Check sheet for the modelled part. Datum: model origin and axes. Units: mm. A direction names the side the tool comes from. Coordinates: 2 decimals unless noted, no trailing zeros. Loops run counter-clockwise (first coordinate to the right, second up) from the corner with the lowest first, then second, coordinate; pieces in that order, holes last. Notation, with made-up numbers: M 80,30 L 87,30 A32 cw 87,64 Z; hole C 17,-38.5 d1. An arc over 180 degrees is marked long. Answer as CSV lines item,"result". Start each with the question number.
from build123d import *

# Parameters (mm, degrees)
CUT_EXTRUDE_1_DEPTH = 3
CHAMFER_1_SIZE      = 0.2


with BuildPart() as part:
    # 草图1 → 旋转1 (revolve)
    with BuildSketch(Plane.YZ, mode=Mode.PRIVATE) as revolve_1_sk:
        Polygon((0, 0), (-4.5, 0), (-4.5, -3.5), (-2.5, -3.5), (-2.5, -38.5), (-2, -38.5), (-2, -45.7), (0, -45.7), align=None)
    revolve(revolve_1_sk.sketch.rotate(Axis((0, 0, -45.7), (0, 0, 1)), 270), axis=Axis((0, 0, -45.7), (0, 0, 1)))

    # 草图2 → 切除-拉伸1 (cut)
    with BuildSketch(Plane.XY):
        Polygon((1.732050808, 0), (0.866025404, 1.5), (-0.866025404, 1.5), (-1.732050808, 0), (-0.866025404, -1.5), (0.866025404, -1.5), align=None)
    extrude(amount=-CUT_EXTRUDE_1_DEPTH, mode=Mode.SUBTRACT)

    # 倒角1
    chamfer_1_edges = [part.edges().sort_by_distance(p)[0] for p in [
        (4.5, 0, -3.5),
        (4.5, 0, 0),
    ]]
    chamfer(chamfer_1_edges, length=CHAMFER_1_SIZE)


solid = part.part
Item 1: Sectioned sample at A-A, the plane x = 0. Record the boundary of the cut face in (y, z), and give its area (3 significant figures).
Item 2: Release check for a two-part mould opening along Y. For faces 1 (the face through (-1.293, 0.76, -1.479)), 2 (the face through (0.54, 2.44, -21.24)), 3 (the face through (-2, 2, -3.5)) record: released by +Y, released by -Y, zero draft, split by the parting line, or undercut.
Item 3: Go/stop test with flat-tipped pins: pin 1 (2 mm diameter, centred on y = -0.5, z = -36.5, fed in from -X); pin 2 (1.5 mm diameter, centred on x = -0.5, y = -0.5, fed in from +Z); pin 3 (3 mm diameter, centred on y = -2.5, z = -29.5, fed in from +X). Record where each tip stops, or that it passes through.
Item 4: Sectioned sample at B-B, the plane z = -7. Record the boundary of the cut face in (x, y), and give its area (3 significant figures).
Item 5: Set-up check for faces 4 (the face through (0, 0, -45.7)), 5 (the face through (1, -2, -38.5)), 6 (the face through (1.305, 0.74, -1.479)): record each of +Z, -Z, +X, -X, +Y, -Y from which the full face is reachable in a straight line by a thin tool's end or side.
Item 6: Material ranges on line 1 (Z direction, x = 1.5, y = 0); line 2 (Z direction, x = 2.25, y = -3); line 3 (Y direction, x = 2, z = -38), recorded low to high. Write a range as from..to.
Reply:
1,outline,"M -4.5,-3.3 L -4.3,-3.5 L -2.5,-3.5 L -2.5,-38.5 L -2,-38.5 L -2,-45.7 L 2,-45.7 L 2,-38.5 L 2.5,-38.5 L 2.5,-3.5 L 4.3,-3.5 L 4.5,-3.3 L 4.5,-0.2 L 4.3,0 L 1.5,0 L 1.5,-3 L -1.5,-3 L -1.5,0 L -4.3,0 L -4.5,-0.2 Z"
1,area,"226 mm²"
2,face 1,"undercut"
2,face 2,"split by the parting line"
2,face 3,"zero draft"
3,pin 1,"x = -2.5"
3,pin 2,"z = -3"
3,pin 3,"x = 2.29"
4,outline,"C 0,0 d5"
4,area,"19.6 mm²"
5,face 4,"-Z, +X, -X, +Y, -Y"
5,face 5,"-Z"
5,face 6,"+Z"
6,line 1,"-45.7..-3"
6,line 2,"-3.5..0"
6,line 3,"-1.5..1.5"
